Geometry check sheet. Reference: the model listing, model coordinates, mm. A direction names the side the tool comes from. Round coordinates to 2 decimals unless told otherwise and drop trailing zeros. Order: outer loops, then holes, each group sorted by start corner. A loop starts at its lowest first (then second) coordinate and runs counter-clockwise, first axis right, second up. Notation, with made-up numbers: M -12.75,18.25 L 12.25,18.25 A31 ccw 12.25,50.25 Z; hole C -1,84 d9. An arc over 180 degrees is marked long. Return JSON: item names as keys, results as strings. Group by question number.
Autodesk Inventor part; units mm, degrees
ref_plane "YZ Plane" through (0, 0, 0) normal (1, 0, 0) x (0, 1, 0)
ref_plane "XZ Plane" through (0, 0, 0) normal (0, 1, 0) x (-1, 0, 0)
ref_plane "XY Plane" through (0, 0, 0) normal (0, 0, 1) x (1, 0, 0)
sketch "Sketch1" plane through (0, 0, 0) normal (0, 0, 1) x (1, 0, 0)
  line L0 (0, 6.16) -> (0, -6.16) construction
  line L1 (-23.38, 0) -> (23.38, 0) construction
  line L2 (16.7, -4.4) -> (-16.7, -4.4)
  line L3 (-16.7, -4.4) -> (-16.7, 4.4)
  line L4 (-16.7, 4.4) -> (16.7, 4.4)
  line L5 (16.7, 4.4) -> (16.7, -4.4)
  line L6 (16.7, -4.4) -> (-16.7, 4.4) construction
  line L7 (-16.7, -4.4) -> (16.7, 4.4) construction
  point P0 (0, 0)
  dimension "d0" = 33.4
  dimension "d1" = 8.8
extrude "Extrusion1" add sketch "Sketch1" along normal mid plane 1.6
sketch "Esquisse2" plane through (0, 0, 0.8) normal (0, 0, 1) x (1, 0, 0)
  line L0 (-16.7, -4.4) -> (16.7, -4.4) construction
  line L1 (16.7, -4.4) -> (16.7, 4.4) construction
  line L2 (16.7, 4.4) -> (-16.7, 4.4) construction
  line L3 (-16.7, 4.4) -> (-16.7, -4.4) construction
  line L4 (0, 8.08) -> (0, -6.48) construction
  line L5 (-23.38, 0) -> (23.38, 0) construction
  line L6 (-14, 4.4) -> (-6, 4.4)
  line L7 (-6, 4.4) -> (-6, 6)
  line L8 (-6, 6) -> (-14, 6)
  line L9 (-14, 6) -> (-14, 4.4)
  line L10 (6, 4.4) -> (14, 4.4)
  line L11 (14, 4.4) -> (14, 6)
  line L12 (14, 6) -> (6, 6)
  line L13 (6, 6) -> (6, 4.4)
  point P0 (0, 0)
  dimension "d4" = 8
  dimension "d5" = 1.6
  dimension "d8" = 20
extrude "Extrusion2" add sketch "Esquisse2" against normal blind 1.6
mirror "Symétrie1" about plane through (0, 0, 0) normal (0, 1, 0) of "Extrusion2"
sketch "Esquisse3" plane through (0, 0, 0.8) normal (0, 0, 1) x (1, 0, 0)
  line L0 (-16.7, -4.4) -> (-14, -4.4) construction
  line L1 (-14, -6) -> (-14, -4.4) construction
  line L2 (-6, -6) -> (-14, -6) construction
  line L3 (-6, -4.4) -> (-6, -6) construction
  line L4 (-6, -4.4) -> (6, -4.4) construction
  line L5 (6, -6) -> (6, -4.4) construction
  line L6 (14, -6) -> (6, -6) construction
  line L7 (14, -4.4) -> (14, -6) construction
  line L8 (14, -4.4) -> (16.7, -4.4) construction
  line L9 (16.7, -4.4) -> (16.7, 4.4) construction
  line L10 (16.7, 4.4) -> (14, 4.4) construction
  line L11 (14, 4.4) -> (14, 6) construction
  line L12 (14, 6) -> (6, 6) construction
  line L13 (6, 6) -> (6, 4.4) construction
  line L14 (6, 4.4) -> (-6, 4.4) construction
  line L15 (-6, 4.4) -> (-6, 6) construction
  line L16 (-6, 6) -> (-14, 6) construction
  line L17 (-14, 6) -> (-14, 4.4) construction
  line L18 (-14, 4.4) -> (-16.7, 4.4) construction
  line L19 (-16.7, 4.4) -> (-16.7, -4.4) construction
  line L20 (-23.38, 0) -> (23.38, 0) construction
  line L21 (0, 8.4) -> (0, -8.4) construction
  line L22 (-16.7, 3) -> (-18.3, 3)
  line L23 (-18.3, 3) -> (-18.3, -3)
  line L24 (-18.3, -3) -> (-16.7, -3)
  line L25 (-16.7, -3) -> (-16.7, 3)
  line L26 (16.7, 3) -> (18.3, 3)
  line L27 (18.3, 3) -> (18.3, -3)
  line L28 (18.3, -3) -> (16.7, -3)
  line L29 (16.7, -3) -> (16.7, 3)
  point P0 (0, 0)
  dimension "d15" = 1.6
  dimension "d16" = 6
extrude "Extrusion3" add sketch "Esquisse3" against normal blind 1.6
properties part number "CaissonCoteBiais" material "PVC-U"
Q1. Section check B-B on z = 0.25. Record the cut outline in (x, y), plus the area to 3 significant figures.
Q2. Material ranges on line 1 along X through (y, z) = (4.75, -0.7); line 2 along Y through (x, z) = (-3.5, 0.45); line 3 along X through (y, z) = (3.75, 0.7), recorded low to high.
Q3. Depth check by flat-ended pin: pin 1 Ø0.8 at (y, z) = (-5, -0.5) entering from +X; pin 2 Ø0.7 at (y, z) = (4, -0.5) entering from +X; pin 3 Ø0.5 at (x, z) = (-15, 0.5) entering from -Y. Enter the tip coordinate at first touch or a pass-through.
Q4. Section check C-C on x = -16. Record the cut outline in (y, z), plus the area to 3 significant figures.
Q5. Release check for a two-part mould opening along X. For faces 5 (the face through (-16.7, -4, 0)), 6 (the face through (-15, 4.4, 0)), 7 (the face through (6, -5, 0)) record: +X half, -X half, draft (parallel to the pull), parting line (faces both ways), or undercut.
Q6. Set-up check for faces 1 (the face through (-14, 5, 0)), 2 (the face through (-6, 5, 0)), 3 (the face through (0, -4.4, 0)), 4 (the face through (-15, -4.4, 0)): record each of +Z, -Z, +X, -X, +Y, -Y from which the full face is reachable in a straight line by a thin tool's end or side.
Q7. Section check A-A on y = -4.75. Record the cut outline in (x, z).
Geometry check:
{
 "1": {"outline": "M -18.3,-3 L -16.7,-3 L -16.7,-4.4 L -14,-4.4 L -14,-6 L -6,-6 L -6,-4.4 L 6,-4.4 L 6,-6 L 14,-6 L 14,-4.4 L 16.7,-4.4 L 16.7,-3 L 18.3,-3 L 18.3,3 L 16.7,3 L 16.7,4.4 L 14,4.4 L 14,6 L 6,6 L 6,4.4 L -6,4.4 L -6,6 L -14,6 L -14,4.4 L -16.7,4.4 L -16.7,3 L -18.3,3 Z", "area": "364 mm^2"},
 "2": {"line 1": "x = -14 to -6, 6 to 14", "line 2": "y = -4.4 to 4.4", "line 3": "x = -16.7 to 16.7"},
 "3": {"pin 1": "stops at x = 14", "pin 2": "stops at x = 16.7", "pin 3": "stops at y = -4.4"},
 "4": {"outline": "M -4.4,-0.8 L 4.4,-0.8 L 4.4,0.8 L -4.4,0.8 Z", "area": "14.1 mm^2"},
 "5": {"face 5": "-X half", "face 6": "draft", "face 7": "undercut"},
 "6": {"face 1": "+Z, -Z, -X, +Y", "face 2": "+Z, -Z, +Y", "face 3": "+Z, -Z, -Y", "face 4": "+Z, -Z, -X, -Y"},
 "7": {"outline": "M -14,-0.8 L -6,-0.8 L -6,0.8 L -14,0.8 Z; M 6,-0.8 L 14,-0.8 L 14,0.8 L 6,0.8 Z"}
}
